from build123d import *

# Parameters (mm, degrees)
SKETCH1_W            = 24.91
SKETCH1_H            = 40.005
BOSS_EXTRUDE1_DEPTH  = 3.175
SKETCH7_W            = 3.175
SKETCH7_H            = 3.175
CUT_EXTRUDE5_DEPTH   = 3.175
LPATTERN2_COUNT      = 6
LPATTERN2_PITCH      = 6.35
LPATTERN2_COUNT_DIR2 = 6
LPATTERN2_PITCH_DIR2 = 6.35
SKETCH8_W            = 3.175
SKETCH8_H            = 0.955
SKETCH8_H_2          = 3.175
CUT_EXTRUDE6_DEPTH   = 3.175
SKETCH9_W            = 3.175
SKETCH9_H            = 3.175
CUT_EXTRUDE7_DEPTH   = 3.175
LPATTERN3_COUNT      = 3
LPATTERN3_PITCH      = 6.35
SKETCH10_W           = 2.685
SKETCH10_H           = 3.175
CUT_EXTRUDE8_DEPTH   = 3.175
SKETCH12_W           = 3.175
SKETCH12_H           = 3.175
BOSS_EXTRUDE2_DEPTH  = 3.175
LPATTERN4_COUNT      = 3
LPATTERN4_PITCH      = 6.35
SKETCH11_R           = 1.5
CUT_EXTRUDE9_DEPTH   = 3.175
LPATTERN5_COUNT      = 3
LPATTERN5_PITCH      = 10


with BuildPart() as part:
    # Sketch1 → Boss-Extrude1 (new body)
    with BuildSketch(Plane.XY):
        with Locations((12.455, 20.0025)):
            Rectangle(SKETCH1_W, SKETCH1_H)
    extrude(amount=BOSS_EXTRUDE1_DEPTH)

    # Sketch7 → Cut-Extrude5 (cut)
    with BuildSketch(Plane(origin=(0, 0, 0), x_dir=(-1, 0, 0), z_dir=(0, 0, -1))):
        with Locations((-1.5875, 31.1125)):
            Rectangle(SKETCH7_W, SKETCH7_H)
    cut_extrude5 = extrude(amount=-CUT_EXTRUDE5_DEPTH, mode=Mode.SUBTRACT)

    # LPattern2: Cut-Extrude5 6 × 6
    with Locations(*[Vector(0, -1, 0) * (i * LPATTERN2_PITCH) + Vector(0, 1, 0) * (j * LPATTERN2_PITCH_DIR2) for i in range(LPATTERN2_COUNT) for j in range(LPATTERN2_COUNT_DIR2) if (i, j) != (0, 0)]):
        add(cut_extrude5, mode=Mode.SUBTRACT)

    # Sketch8 → Cut-Extrude6 (cut)
    with BuildSketch(Plane(origin=(0, 0, 0), x_dir=(-1, 0, 0), z_dir=(0, 0, -1))):
        with Locations((-1.5875, 39.5275)):
            Rectangle(SKETCH8_W, SKETCH8_H)
        with Locations((-1.5875, 2.5375)):
            Rectangle(SKETCH8_W, SKETCH8_H_2)
    extrude(amount=-CUT_EXTRUDE6_DEPTH, mode=Mode.SUBTRACT)

    # Sketch9 → Cut-Extrude7 (cut)
    with BuildSketch(Plane(origin=(0, 0, 0), x_dir=(-1, 0, 0), z_dir=(0, 0, -1))):
        with Locations((-20.1475, 1.5875)):
            Rectangle(SKETCH9_W, SKETCH9_H)
    cut_extrude7 = extrude(amount=-CUT_EXTRUDE7_DEPTH, mode=Mode.SUBTRACT)

    # LPattern3: Cut-Extrude7 ×3
    with Locations(*[(-i * LPATTERN3_PITCH, 0, 0) for i in range(1, LPATTERN3_COUNT)]):
        add(cut_extrude7, mode=Mode.SUBTRACT)

    # Sketch10 → Cut-Extrude8 (cut)
    with BuildSketch(Plane(origin=(0, 0, 0), x_dir=(-1, 0, 0), z_dir=(0, 0, -1))):
        with Locations((-4.5175, 1.5875)):
            Rectangle(SKETCH10_W, SKETCH10_H)
    extrude(amount=-CUT_EXTRUDE8_DEPTH, mode=Mode.SUBTRACT)

    # Sketch12 → Boss-Extrude2 (add)
    with BuildSketch(Plane(origin=(0, 0, 0), x_dir=(-1, 0, 0), z_dir=(0, 0, -1))):
        with Locations((-23.3225, 41.5925)):
            Rectangle(SKETCH12_W, SKETCH12_H)
    boss_extrude2 = extrude(amount=-BOSS_EXTRUDE2_DEPTH)

    # LPattern4: Boss-Extrude2 ×3
    with Locations(*[(-i * LPATTERN4_PITCH, 0, 0) for i in range(1, LPATTERN4_COUNT)]):
        add(boss_extrude2)

    # Sketch11 → Cut-Extrude9 (cut)
    with BuildSketch(Plane(origin=(0, 0, 0), x_dir=(-1, 0, 0), z_dir=(0, 0, -1))):
        with Locations((-15.63, 31.589068697)):
            Circle(SKETCH11_R)
    cut_extrude9 = extrude(amount=-CUT_EXTRUDE9_DEPTH, mode=Mode.SUBTRACT)

    # LPattern5: Cut-Extrude9 ×3
    with Locations(*[(0, -i * LPATTERN5_PITCH, 0) for i in range(1, LPATTERN5_COUNT)]):
        add(cut_extrude9, mode=Mode.SUBTRACT)


solid = part.part
Could you check a few things on this model? Use its own coordinates, in mm. A direction names the side the tool comes from. Give positions to 0.01 mm unless a question says otherwise; leave off trailing zeros. Loops run counter-clockwise (first coordinate to the right, second up) from the corner with the lowest first, then second, coordinate; pieces in that order, holes last. Notation, with made-up numbers: M 35,57 L 51,57 A5 ccw 51,62 Z; hole C 32.25,33.5 d10. An arc over 180 degrees is marked long. Answer as a JSON object with one key per item and string values.
Q1. If I drill on probe 1 along Y at (x, z) = (15.63, 0.9); probe 2 along X at (y, z) = (11.5, 1) (3 decimals); probe 3 along X at (y, z) = (5, 1.7) (3 decimals), over which ranges is the centre line in solid material (lowest first)? Write a range as [from, to].
Values found:
{"probe 1": "y = [0, 10.09], [13.09, 20.09], [23.09, 30.09], [33.09, 43.18]", "probe 2": "x = [3.175, 14.133], [17.127, 24.91]", "probe 3": "x = [3.175, 24.91]"}
Q2. If we mould it in two halves opening along X, with no side actions, what happens to faces 6 (the flat face through (3.175, 38, 2)), 7 (the flat face through (18.56, 42, 2)), 8 (the cylindrical face through (14.2, 32.04, 1.57)), 9 (the flat face through (24.91, 21, 2))? For each: pulls with the +X half, pulls with the -X half, needs draft (parallel to the pull), parting line crosses it, or undercut.
Values found:
{"face 6": "pulls with the -X half", "face 7": "undercut", "face 8": "undercut", "face 9": "pulls with the +X half"}
Q3. Suppose I cut it at D-D, the plane z = 0.9. State how many separate pieces and enclosed holes the cut face has, plus the area to 3 significant figures.
Values found:
{"separate pieces": "1", "enclosed holes": "3", "area": "890 mm²"}
Q4. Suppose I cut it at A-A, the plane y = 11. List the corners of the cut face in (x, z) for me (1 decimal).
Values found:
{"outline": "M 3.2,0 L 14.3,0 L 14.3,3.2 L 3.2,3.2 Z; M 17,0 L 24.9,0 L 24.9,3.2 L 17,3.2 Z"}
Q5. For faces 1 (the flat face through (21.735, 2, 2)), 2 (the flat face through (12.21, 42, 2)), 3 (the flat face through (3.175, 18, 2)), 4 (the flat face through (6, 40.005, 2)), 5 (the flat face through (6, 3.175, 2)), which set-ups out of +Z, -Z, +X, -X, +Y, -Y let a thin tool reach every point of the face, with its end or its side?
Values found:
{"face 1": "+Z, -Z, -Y", "face 2": "+Z, -Z, +Y", "face 3": "+Z, -Z, -X", "face 4": "+Z, -Z, -X, +Y", "face 5": "+Z, -Z, -X, -Y"}
Q6. Suppose I cut it at C-C, the plane y = 17.5. List the corners of the cut face in (x, z) for me (3 decimals).
Values found:
{"outline": "M 3.175,0 L 24.91,0 L 24.91,3.175 L 3.175,3.175 Z"}
Q7. Suppose I cut it at B-B, the plane x = 21.25. List the corners of the cut face in (y, z) for me (3 decimals), plus the area to 3 significant figures.
Values found:
{"outline": "M 3.175,0 L 40.005,0 L 40.005,3.175 L 3.175,3.175 Z", "area": "117 mm²"}
Q8. For P1, Ø1, axis at y = 1, z = 2, coming from the -X side (3 decimals); P2, Ø1.6, axis at x = 2, z = 2, coming from the -Y side; P3, Ø3.5, axis at x = 15.63, y = 11.59, coming from the -Z side; P4, Ø1, axis at y = 12, z = 1.5, coming from the -X side (3 decimals), each with a flat end and sliding along its axis, tell me the tip position at first contact or that it passes through.
Values found:
{"P1": "stops at x = 9.035", "P2": "stops at y = 7.3", "P3": "stops at z = 0", "P4": "stops at x = 3.175"}
